from build123d import *

# Parameters (mm, degrees)
BASE_FLANGE1_DEPTH            = 1.1
EDGE_FLANGE1_STRIP_W          = 5.8732
EDGE_FLANGE1_STRIP_H          = 1.1
EDGE_FLANGE1_STRIP_CUT_DEPTH  = 9.1
EDGE_FLANGE1_RELIEF_W         = 6.4232
EDGE_FLANGE1_RELIEF_H         = 0.55
EDGE_FLANGE1_RELIEF_CUT_DEPTH = 1.1
EDGE_FLANGE1_DEPTH            = 9.1
EDGE_FLANGE2_STRIP_W          = 5.8732
EDGE_FLANGE2_STRIP_H          = 1.1
EDGE_FLANGE2_STRIP_CUT_DEPTH  = 9.1
EDGE_FLANGE2_DEPTH            = 9.1
SKETCH9_R                     = 1.65
EXTRUDE1_DEPTH                = 1.1
SKETCHED_START                = -30
SKETCHED_BEND2_DEPTH          = 58.1
SKETCHED_BEND2_2_OUTLINE_W    = 51.994658845
SKETCHED_BEND2_2_OUTLINE_H    = 1.1
SKETCHED_BEND2_2_DEPTH        = 58.1
SKETCHED_START_2              = -20
SKETCHED_BEND2_3_DEPTH        = 48.1
SKETCHED_BEND6_DEPTH          = 58.1
SKETCHED_BEND6_2_DEPTH        = 58.1


# Read off the part's stored shape, not the designer's step: Sketched Bend2, Sketched Bend6
# Sheet-metal steps are written as plain solids
with BuildPart() as part:
    # Sketch1 → Base-Flange1 (new body)
    with BuildSketch(Plane(origin=(0, 0, 0), x_dir=(1, 0, 0), z_dir=(0, 1, 0))):
        with BuildLine():
            Line((-30.1, 1.2), (-21, 1.2))
            Line((-21, 1.2), (-21, -0.6))
            Line((-21, -0.6), (-20, -0.6))
            Line((-20, -0.6), (-20, 24.411105723))
            Line((-20, 24.411105723), (-30, 24.411105723))
            Line((-30, 24.411105723), (-30, 76.405764568))
            Line((-30, 76.405764568), (28.1, 76.405764568))
            Line((28.1, 76.405764568), (28.1, 19.7))
            Line((28.1, 19.7), (28.1, -4.05))
            ThreePointArc((28.1, -4.05), (26.928427125, -6.878427125), (24.1, -8.05))
            Line((24.1, -8.05), (18.1, -8.05))
            ThreePointArc((18.1, -8.05), (14.863529932, -15.863529932), (7.05, -19.1))
            Line((7.05, -19.1), (-10.1, -19.1))
            ThreePointArc((-10.1, -19.1), (-16.605382387, -16.405382387), (-19.3, -9.9))
            Line((-19.3, -9.9), (-26.1, -9.9))
            ThreePointArc((-26.1, -9.9), (-28.928427125, -8.728427125), (-30.1, -5.9))
            Line((-30.1, -5.9), (-30.1, 1.2))
        make_face()
    extrude(amount=BASE_FLANGE1_DEPTH)

    # Edge-Flange1 strip (across the edge) → Edge-Flange1 strip cut (cut)
    with BuildSketch(Plane(origin=(-21, 1.1, -1.2), x_dir=(0, 0, 1), z_dir=(-1, 0, 0))):
        with Locations((-1.1, -0.55)):
            Rectangle(EDGE_FLANGE1_STRIP_W, EDGE_FLANGE1_STRIP_H)
    extrude(amount=EDGE_FLANGE1_STRIP_CUT_DEPTH, mode=Mode.SUBTRACT)

    # Edge-Flange1 relief (on the sheet) → Edge-Flange1 relief cut (cut)
    with BuildSketch(Plane(origin=(-21, 1.1, 0.6366), x_dir=(0, 0, 1), z_dir=(0, 1, 0))):
        with Locations((-2.6616, 0.275)):
            Rectangle(EDGE_FLANGE1_RELIEF_W, EDGE_FLANGE1_RELIEF_H)
    extrude(amount=-EDGE_FLANGE1_RELIEF_CUT_DEPTH, mode=Mode.SUBTRACT)

    # Edge-Flange1 section (across the edge) → Edge-Flange1 (add)
    with BuildSketch(Plane(origin=(-21, 1.1, -1.2), x_dir=(0, 0, 1), z_dir=(-1, 0, 0))):
        with BuildLine():
            Line((0, 0.7366), (0, 5.8))
            Line((0, 5.8), (1.1, 5.8))
            Line((1.1, 5.8), (1.1, 0.7366))
            ThreePointArc((1.1, 0.7366), (1.315745145, 0.215745145), (1.8366, 0))
            Line((1.8366, 0), (1.8366, -1.1))
            ThreePointArc((1.8366, -1.1), (0.537927686, -0.562072314), (0, 0.7366))
        make_face()
    extrude(amount=EDGE_FLANGE1_DEPTH)

    # Edge-Flange2 strip (across the edge) → Edge-Flange2 strip cut (cut)
    with BuildSketch(Plane(origin=(-30.1, 6.9, -1.2), x_dir=(0, -1, 0), z_dir=(1, 0, 0))):
        with Locations((-1.1, -0.55)):
            Rectangle(EDGE_FLANGE2_STRIP_W, EDGE_FLANGE2_STRIP_H)
    extrude(amount=EDGE_FLANGE2_STRIP_CUT_DEPTH, mode=Mode.SUBTRACT)

    # Edge-Flange2 section (across the edge) → Edge-Flange2 (add)
    with BuildSketch(Plane(origin=(-30.1, 6.9, -1.2), x_dir=(0, -1, 0), z_dir=(1, 0, 0))):
        with BuildLine():
            Line((0, 0.7366), (0, 8.2))
            Line((0, 8.2), (1.1, 8.2))
            Line((1.1, 8.2), (1.1, 0.7366))
            ThreePointArc((1.1, 0.7366), (1.315745145, 0.215745145), (1.8366, 0))
            Line((1.8366, 0), (1.8366, -1.1))
            ThreePointArc((1.8366, -1.1), (0.537927686, -0.562072314), (0, 0.7366))
        make_face()
    extrude(amount=EDGE_FLANGE2_DEPTH)

    # Sketch9 → Extrude1 (cut)
    with BuildSketch(Plane(origin=(0, 6.9, 0), x_dir=(1, 0, 0), z_dir=(0, 1, 0))):
        with Locations(Location((-25.55, 6.05, 0), (0, 0, 270))):
            Circle(SKETCH9_R)
        with BuildLine():
            Line((-30.1, 6.4), (-30.1, 9.4))
            Line((-30.1, 9.4), (-27.1, 9.4))
            ThreePointArc((-27.1, 9.4), (-29.221320344, 8.521320344), (-30.1, 6.4))
        make_face()
        with BuildLine():
            Line((-24, 9.4), (-21, 9.4))
            Line((-21, 9.4), (-21, 6.4))
            ThreePointArc((-21, 6.4), (-21.878679656, 8.521320344), (-24, 9.4))
        make_face()
    extrude(amount=-EXTRUDE1_DEPTH, mode=Mode.SUBTRACT)

    # Sketched Bend2 outline → Sketched Bend2 (cut)
    with BuildSketch(Plane.YZ.offset(SKETCHED_START)):
        with BuildLine():
            ThreePointArc((1.1, -19.495814944), (0.299404636, -18.818452246), (-1.2e-08, -17.8134))
            Line((-1.2e-08, -17.8134), (0, -76.405764568))
            Line((0, -76.405764568), (1.1, -76.405764568))
            Line((1.1, -76.405764568), (1.1, -19.495814944))
        make_face()
    extrude(amount=SKETCHED_BEND2_DEPTH, mode=Mode.SUBTRACT)



with BuildPart() as body_2:
    # Sketched Bend2 2 outline → Sketched Bend2 2 (new body)
    with BuildSketch(Plane.YZ.offset(SKETCHED_START)):
        with Locations((32.410648591, -19.1)):
            Rectangle(SKETCHED_BEND2_2_OUTLINE_W, SKETCHED_BEND2_2_OUTLINE_H)
    extrude(amount=SKETCHED_BEND2_2_DEPTH)


with BuildPart() as part_1:
    add(part.part)

    add(body_2.part)  # Sketched Bend2 3 merges body 2
    # Sketched Bend2 3 outline → Sketched Bend2 3 (add)
    with BuildSketch(Plane.YZ.offset(SKETCHED_START_2)):
        with BuildLine():
            Line((6.413319169, -18.55), (1.836600012, -18.550000012))
            ThreePointArc((1.836600012, -18.550000012), (1.315745141, -18.334254868), (1.099999988, -17.8134))
            Line((1.099999988, -17.8134), (1.1, -19.495814944))
            ThreePointArc((1.1, -19.495814944), (1.460317993, -19.611040525), (1.8366, -19.650000012))
            Line((1.8366, -19.650000012), (6.413319169, -19.65))
            Line((6.413319169, -19.65), (6.413319169, -18.55))
        make_face()
    extrude(amount=SKETCHED_BEND2_3_DEPTH)

    # Sketched Bend6 outline → Sketched Bend6 (cut)
    with BuildSketch(Plane.YZ.offset(SKETCHED_START)):
        with BuildLine():
            Line((58.407978014, -18.55), (7.9634, -18.549999994))
            ThreePointArc((7.9634, -18.549999994), (8.968452241, -18.849404641), (9.645814937, -19.65))
            Line((9.645814937, -19.65), (58.407978014, -19.65))
            Line((58.407978014, -19.65), (58.407978014, -18.55))
        make_face()
    extrude(amount=SKETCHED_BEND6_DEPTH, mode=Mode.SUBTRACT)

    # Sketched Bend6 2 outline → Sketched Bend6 2 (add)
    with BuildSketch(Plane.YZ.offset(SKETCHED_START)):
        with BuildLine():
            ThreePointArc((9.800000006, -20.3866), (9.761040518, -20.010317993), (9.645814937, -19.65))
            Line((9.645814937, -19.65), (7.9634, -19.649999994))
            ThreePointArc((7.9634, -19.649999994), (8.484254859, -19.865745141), (8.700000006, -20.3866))
            Line((8.700000006, -20.3866), (8.7, -68.81019146))
            Line((8.7, -68.81019146), (9.8, -68.81019146))
            Line((9.8, -68.81019146), (9.800000006, -20.3866))
        make_face()
    extrude(amount=SKETCHED_BEND6_2_DEPTH)


solid = part_1.part
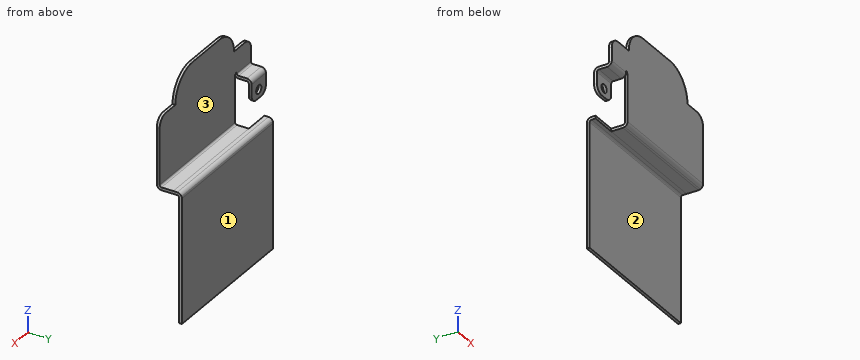
The listing builds one solid part. Answer for the finished solid, in the listing's coordinates (mm). Face numbers are marked on the shaded views. A direction names the side the tool comes from. Give positions to 0.01 mm unless a question says otherwise; leave off trailing zeros. Loops run counter-clockwise (first coordinate to the right, second up) from the corner with the lowest first, then second, coordinate; pieces in that order, holes last. Notation, with made-up numbers: (75.25, 3.5) - (116.25, 3.5) arc R16 cw to (116.25, 29.5) - close; hole circle Ø1 at (66.5, 70.5). An arc over 180 degrees is marked (long way). Use one line per item in the form item = value.
1. Section D-D on z = -39 is taken. Give the vertices of the cut face in (x, y).
Calculated:
outline = (-30, 8.7) - (28.1, 8.7) - (28.1, 9.8) - (-30, 9.8) - close
2. Section C-C on x = -22.5 is taken. Give the vertices of the cut face in (y, z).
Calculated:
outline = (0, 0.64) arc R1.84 ccw to (1.84, -1.2) - (5.06, -1.2) arc R0.74 cw to (5.8, -1.94) - (5.8, -9) - (6.9, -9) - (6.9, -1.94) arc R1.84 ccw to (5.06, -0.1) - (1.84, -0.1) arc R0.74 cw to (1.1, 0.64) - (1.1, 9.9) - (0, 9.9) - close; (6.41, -19.65) - (7.96, -19.65) arc R0.74 cw to (8.7, -20.39) - (8.7, -68.81) - (9.8, -68.81) - (9.8, -20.39) arc R1.84 ccw to (7.96, -18.55) - (6.41, -18.55) - close
3. Given pin 1 Ø0.6 at (x, z) = (-22.5, -19) entering from -Y; pin 2 Ø1.2 at (x, y) = (-26, 6.5) entering from -Z; pin 3 Ø0.9 at (x, y) = (21.5, 1) entering from +Z, each flat-ended and moving along its own axis, determine where each tip first touches the part or whether it passes through.
Calculated:
pin_1 = 6.41
pin_2 = -19.65
pin_3 = 8.05
4. Which of the six approach directions +Z, -Z, +X, -X, +Y, -Y give full straight-line access (tool end or side, diameter ignored) to the marked faces 1, 2 and 3?
Calculated:
face_1 = +Z, -Z, +X, -X, +Y
face_2 = -Z, +X, -X, -Y
face_3 = +Z, +X, +Y
5. Section B-B on z = -3.5 is taken. Give the vertices of the cut face in (x, y).
Calculated:
outline = (-30.1, 5.8) - (-21, 5.8) - (-21, 6.9) - (-30.1, 6.9) - close; (-20, 0) - (28.1, 0) - (28.1, 1.1) - (-20, 1.1) - close
6. Section A-A on y = 3.25 is taken. Give the vertices of the cut face in (x, z).
Calculated:
outline = (-30.1, -1.2) - (-21, -1.2) - (-21, -0.1) - (-30.1, -0.1) - close; (-20, -19.65) - (28.1, -19.65) - (28.1, -18.55) - (-20, -18.55) - close
7. Find the intervals of material crossed by line 1 along X through (y, z) = (6.55, -6.05); line 2 along Y through (x, z) = (-20, -65); line 3 along X through (y, z) = (4, -19), in increasing order. Write a range as [from, to].
Calculated:
line_1 = [-30.1, -27.2], [-23.9, -21]
line_2 = [8.7, 9.8]
line_3 = [-20, 28.1]
